from build123d import *

# Parameters (mm, degrees)
BOSS_EXTRUDE1_DEPTH      = 10
BOSS_EXTRUDE1_DEPTH_BACK = 10
CUT_EXTRUDE1_DEPTH       = 5
CUT_EXTRUDE1_DEPTH_BACK  = 5
SKETCH4_R                = 3.75
BOSS_EXTRUDE2_DEPTH      = 25
SKETCH5_R                = 3.75
CUT_EXTRUDE3_DEPTH       = 25


with BuildPart() as part:
    # Sketch1 → Boss-Extrude1 (new, two sides: drawn at the far end of the back side and taken through both)
    with BuildSketch(Plane.XY.offset(-BOSS_EXTRUDE1_DEPTH_BACK)):
        with BuildLine():
            Line((-55, -10), (-50, -10))
            Line((-50, -10), (-50, 0))
            ThreePointArc((-50, 0), (0, 50), (50, 0))
            Line((50, 0), (50, -10))
            Line((50, -10), (55, -10))
            Line((55, -10), (55, 0))
            ThreePointArc((55, 0), (0, 55), (-55, 0))
            Line((-55, 0), (-55, -10))
        make_face()
    extrude(amount=BOSS_EXTRUDE1_DEPTH + BOSS_EXTRUDE1_DEPTH_BACK)

    # Sketch2 → Cut-Extrude1 (cut, two sides: drawn at the far end of the back side and taken through both)
    with BuildSketch(Plane.XY.offset(-CUT_EXTRUDE1_DEPTH_BACK)):
        with BuildLine():
            Line((0, 0), (-54.164426416, 9.550649772))
            ThreePointArc((-54.164426416, 9.550649772), (0, 55), (54.164426416, 9.550649772))
            Line((54.164426416, 9.550649772), (0, 0))
        make_face()
    extrude(amount=CUT_EXTRUDE1_DEPTH + CUT_EXTRUDE1_DEPTH_BACK, mode=Mode.SUBTRACT)

    # Sketch4 → Boss-Extrude2 (add)
    with BuildSketch(Plane.ZY.offset(55)):
        Circle(SKETCH4_R)
    extrude(amount=BOSS_EXTRUDE2_DEPTH)

    # Sketch5 → Cut-Extrude3 (cut)
    with BuildSketch(Plane(origin=(55, 0, 0), x_dir=(0, 0, -1), z_dir=(1, 0, 0))):
        with Locations(Location((0, 0, 0), (0, 0, 180))):
            Circle(SKETCH5_R)
    extrude(amount=-CUT_EXTRUDE3_DEPTH, mode=Mode.SUBTRACT)


solid = part.part
Verification items for the finished model (mm, model axes). A direction names the side the tool comes from. Coordinates: 2 decimals unless noted, no trailing zeros. Order: outer loops, then holes, each group sorted by start corner. A loop starts at its lowest first (then second) coordinate and runs counter-clockwise, first axis right, second up. Notation, with made-up numbers: M 73.25,32.25 L 78.25,32.25 A14 cw 78.25,57.25 Z; hole C 19.25,-19.75 d8. An arc over 180 degrees is marked long. One line per item, written item: value. Start each with the question number.
Item 1: Sectioned sample at B-B (y = 39). Enter the section's corners in (x, z).
Item 2: Sectioned sample at C-C (z = 1.5). Enter the section's corners in (x, y).
Item 3: Access from +Z, -Z, +X, -X, +Y, -Y to the whole of each face (thin tool, end or side, straight path). Record for faces 1 (the cylindrical face through (-67.325, 0.165, -3.746)), 2 (the flat face through (-51.67, 9.11, -0.07)), 3 (the flat face through (-50, -5, 0)), 4 (the cylindrical face through (52.47, -3.16, 2.02)).
Item 4: Sectioned sample at D-D (z = -8.5). Enter the section's corners in (x, y).
Item 5: Sectioned sample at A-A (x = 0). Enter the section's corners in (y, z).
Item 6: Mould release check, pull along X, two halves, no side actions. Record for faces 5 (the flat face through (50, -5, 0)), 6 (the flat face through (-55, -5, 0)), 7 (the flat face through (-53, -10, 0)), 8 (the flat face through (55, -5, 0)): released by +X, released by -X, zero draft, split by the parting line, or undercut.
Item 7: Gauge pin test, flat ends, axial feed: pin 1 (3 mm diameter, centred on y = 3, z = 0, fed in from +X); pin 2 (6 mm diameter, centred on y = 47, z = -5, fed in from +X); pin 3 (8 mm diameter, centred on y = 11.5, z = -2.5, fed in from +X). Record the tip position at first contact, or that the pin passes through.
Item 8: Scan lines: probe 1 along X at (y, z) = (-6, -8.5); probe 2 along Z at (x, y) = (-39, 33); probe 3 along X at (y, z) = (-1, 2.75). Record each from-to range of solid material in increasing order.
Conclusion:
1. outline: M -38.78,-10 L -31.29,-10 L -31.29,-5 L -38.78,-5 Z; M -38.78,5 L -31.29,5 L -31.29,10 L -38.78,10 Z; M 31.29,-10 L 38.78,-10 L 38.78,-5 L 31.29,-5 Z; M 31.29,5 L 38.78,5 L 38.78,10 L 31.29,10 Z
2. outline: M -80,-3.44 L -55,-3.44 L -55,-10 L -50,-10 L -50,0 A50 cw -49.24,8.68 L -54.16,9.55 A55 ccw -55,0 L -55,3.44 L -80,3.44 Z; M 49.24,8.68 A50 cw 49.88,3.44 L 54.89,3.44 A55 ccw 54.16,9.55 Z; M 50,-10 L 55,-10 L 55,-3.44 L 50,-3.44 Z
3. face 1: -X
3. face 2: +Y
3. face 3: +Z, -Z, -Y
3. face 4: +X
4. outline: M -55,-10 L -50,-10 L -50,0 A50 cw 50,0 L 50,-10 L 55,-10 L 55,0 A55 ccw -55,0 Z
5. outline: M 50,-10 L 55,-10 L 55,-5 L 50,-5 Z; M 50,5 L 55,5 L 55,10 L 50,10 Z
6. face 5: undercut
6. face 6: released by -X
6. face 7: zero draft
6. face 8: released by +X
7. pin 1: stops at x = 54.89
7. pin 2: stops at x = 33
7. pin 3: stops at x = 54.49
8. probe 1: x = -55 to -50, 50 to 55
8. probe 2: z = -10 to -5, 5 to 10
8. probe 3: x = -80 to -50
